Geometry: final body of the model. Coordinates: model frame, mm. Give positions to 0.01 mm unless a question says otherwise; leave off trailing zeros. Loops run counter-clockwise (first coordinate to the right, second up) from the corner with the lowest first, then second, coordinate; pieces in that order, holes last. Notation, with made-up numbers: (-36, 5.25) -> (-29, 5.25) arc R30 ccw to (-29, 33.25) -> close; hole circle Ø6 at (72.5, 84). An arc over 180 degrees is marked (long way). Answer in a Markdown table with one row per item. Add a question column.
from build123d import *

# Parameters (mm, degrees)
SKETCH1_R           = 58.5
BOSS_EXTRUDE2_DEPTH = 100
SKETCH3_R           = 48.5
CUT_EXTRUDE1_DEPTH  = 20
FILLET1_R           = 1
CHAMFER1_SIZE       = 4
FILLET3_R           = 2
FILLET4_R           = 10


with BuildPart() as part:
    # Sketch1 → Boss-Extrude2 (new body)
    with BuildSketch(Plane.XY):
        Circle(SKETCH1_R)
    extrude(amount=BOSS_EXTRUDE2_DEPTH)

    # Sketch3 → Cut-Extrude1 (cut)
    with BuildSketch(Plane.XY.offset(100)):
        Circle(SKETCH3_R)
    extrude(amount=-CUT_EXTRUDE1_DEPTH, mode=Mode.SUBTRACT)

    # Fillet1
    fillet1_edges = [part.edges().sort_by_distance(p)[0] for p in [
        (-48.5, 0, 100),
    ]]
    fillet(fillet1_edges, radius=FILLET1_R)

    # Chamfer1
    chamfer1_edges = [part.edges().sort_by_distance(p)[0] for p in [
        (-58.5, 0, 100),
    ]]
    chamfer(chamfer1_edges, length=CHAMFER1_SIZE)

    # Fillet3
    fillet3_edges = [part.edges().sort_by_distance(p)[0] for p in [
        (-54.5, 0, 100),
        (-58.5, 0, 96),
    ]]
    fillet(fillet3_edges, radius=FILLET3_R)

    # Fillet4
    fillet4_edges = [part.edges().sort_by_distance(p)[0] for p in [
        (-58.5, 0, 0),
    ]]
    fillet(fillet4_edges, radius=FILLET4_R)


solid = part.part
(1) Draft query along Y for faces 1 (the flat face through (-1, 1, 0)), 2 (the cylindrical face through (22.38, -43.028, 89.633)), 3 (the conical face through (25.5, -49.028, 99.237)), 4 (the flat face through (-1, 1, 80)). Return one class per face: +Y half, -Y half, draft (parallel to the pull), parting line (faces both ways), or undercut.
(2) Material intervals for line 1 along Y through (x, z) = (0, 89.25); line 2 along Z through (x, y) = (-31, 4); line 3 along Y through (x, z) = (-0.5, 46), sorted ascending. Write a range as from..to.
(3) Pin query (flat end, axial travel): pin 1 Ø6 at (x, y) = (-46.5, -34) entering from +Z; pin 2 Ø1.5 at (x, z) = (39, 58) entering from +Y; pin 3 Ø3 at (x, y) = (-17.5, 7.5) entering from +Z. Return the tip coordinate at first contact, or that it passes through.
(4) Cut plane A-A on z = 76.5. Return the cut outline in (x, y), then the cut area to 3 significant figures.
Answer list:
| question | item | result |
|---|---|---|
| 1 | face 1 | draft |
| 1 | face 2 | undercut |
| 1 | face 3 | parting line |
| 1 | face 4 | undercut |
| 2 | line 1 | y = -58.5..-48.5, 48.5..58.5 |
| 2 | line 2 | z = 0..80 |
| 2 | line 3 | y = -58.5..58.5 |
| 3 | pin 1 | stops at z = 99.77 |
| 3 | pin 2 | stops at y = 44.26 |
| 3 | pin 3 | stops at z = 80 |
| 4 | outline | circle Ø117 at (0, 0) |
| 4 | area | 10,800 mm² |
